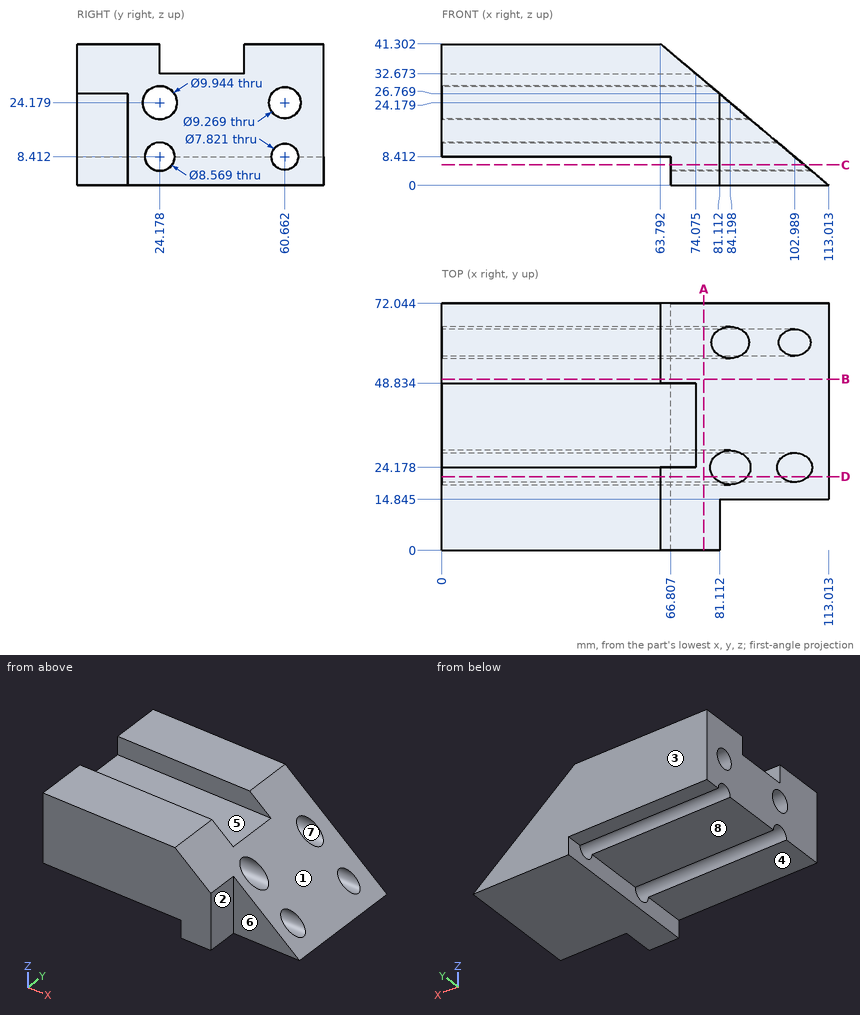
Input: dimensioned drawing with shaded views. Units: mm. Origin: part minimum x, y, z. A direction names the side the tool comes from. Coordinates: 2 decimals unless noted, no trailing zeros. Write each loop counter-clockwise with the first axis right and the second up, starting at its lowest first coordinate (ties: lowest second). Pieces come first, ordered by that corner, then holes. Notation, with made-up numbers: M -14.5,25 L 8.5,25 A29 cw 8.5,63 Z; hole C 24,33 d8. An arc over 180 degrees is marked long. Use a Markdown table: item, result.
1) Section D-D, the plane y = 21.5. Output: boundary loops of the cut face in (x, z) (1 decimal), then the cut area to 3 significant figures.
Conclusion:
| item | result |
|---|---|
| outline | M 0,11.8 L 99,11.8 L 89.2,20 L 0,20 Z; M 0,28.4 L 79.2,28.4 L 63.8,41.3 L 0,41.3 Z; M 66.8,0 L 113,0 L 107,5.1 L 66.8,5.1 Z |
| area | 1,920 mm^2 |
2) First-contact query: pin 1 Ø1.5 at (y, z) = (47.5, 9) entering from +X; pin 2 Ø1.5 at (x, y) = (45.5, 34.5) entering from +Z; pin 3 Ø12 at (y, z) = (42.5, 11.5) entering from +X. Flat tips, straight axial feed; report the tip coordinate or a pass-through.
Conclusion:
| item | result |
|---|---|
| pin 1 | stops at x = 103.18 |
| pin 2 | stops at z = 32.67 |
| pin 3 | stops at x = 106.46 |
3) Reachability of the marked faces 1, 2, 3, 4 and 5 from +Z, -Z, +X, -X, +Y, -Y: full face, straight path, thin tool, end or side. Return the list, or none.
Conclusion:
| item | result |
|---|---|
| face 1 | +Z, +X, +Y, -Y |
| face 2 | +Z, -Z, +X, -Y |
| face 3 | +Z, -Z, +X, -X, +Y |
| face 4 | -Z, -X, +Y, -Y |
| face 5 | +Z, +X, -X |
4) Section C-C, the plane z = 6. Output: boundary loops of the cut face in (x, y) (1 decimal).
Conclusion:
| item | result |
|---|---|
| outline | M 66.8,0 L 81.1,0 L 81.1,14.8 L 105.9,14.8 L 105.9,20.6 L 66.8,20.6 Z; M 66.8,27.7 L 105.9,27.7 L 105.9,57.6 L 66.8,57.6 Z; M 66.8,63.7 L 105.9,63.7 L 105.9,72 L 66.8,72 Z |
5) Section A-A, the plane x = 76.5. Output: boundary loops of the cut face in (y, z) (1 decimal), then the cut area to 3 significant figures.
Conclusion:
| item | result |
|---|---|
| outline | M 0,0 L 72,0 L 72,30.6 L 0,30.6 Z; hole C 24.2,24.2 d9.9; hole C 24.2,8.4 d8.6; hole C 60.7,24.2 d9.3; hole C 60.7,8.4 d7.8 |
| area | 1,960 mm^2 |
6) Mould query, pull axis Y, two halves, no side actions, for the marked faces 6, 7 and 8. Classes: pulls with the +Y half, pulls with the -Y half, needs draft (parallel to the pull), parting line crosses it, or undercut.
Conclusion:
| item | result |
|---|---|
| face 6 | pulls with the -Y half |
| face 7 | undercut |
| face 8 | needs draft |
7) Ray query, L1, parallel to Y at x = 29.5, z = 33; L2, parallel to Z at x = 34.5, y = 7; L3, parallel to Y at x = 86.5, z = 2.5 (1 decimal). Return the intervals inside material, ascending.
Conclusion:
| item | result |
|---|---|
| L1 | y = 0 to 24.18, 48.83 to 72.04 |
| L2 | z = 8.41 to 41.3 |
| L3 | y = 14.8 to 72 |
8) Section B-B, the plane y = 50. Output: boundary loops of the cut face in (x, z).
Conclusion:
| item | result |
|---|---|
| outline | M 0,8.41 L 66.81,8.41 L 66.81,0 L 113.01,0 L 63.79,41.3 L 0,41.3 Z |
